Design review of the part built by this model. Coordinates are the model's own, in mm. A direction names the side the tool comes from. Round coordinates to 2 decimals unless told otherwise and drop trailing zeros. Loops run counter-clockwise (first coordinate to the right, second up) from the corner with the lowest first, then second, coordinate; pieces in that order, holes last. Notation, with made-up numbers: (39.25, -29.75) - (49.25, -29.75) arc R26 cw to (49.25, -3.75) - close; hole circle Ø3 at (31.25, 23.5). An arc over 180 degrees is marked (long way). Answer as CSV lines item,"result". Start each with the question number.
(1) For P1, Ø1.5, axis at x = 0.5, y = 2, coming from the +Z side; P2, Ø1, axis at x = 1.5, z = 3, coming from the +Y side; P3, Ø1.5, axis at x = 1.5, y = -1, coming from the -Z side, all flat-tipped, find the tip position at first contact; note any pin that passes through.
(2) Wall thickness on L1, parallel to X at y = -0.6, z = -2; L2, parallel to Y at x = -0.05, z = 2.25; L3, parallel to Z at x = 0, y = 1.55: over which ranges is each line inside the solid? List them lowest first.
(3) For faces 4 (the flat face through (0, 0, 5)), 5 (the cylindrical face through (-1.5, 0.07, 2.46)), list the 3-axis set-ups (+Z, -Z, +X, -X, +Y, -Y) from which the entire face can be reached by the end or side of a thin tool; tool diameter is ignored.
(4) Consider section C-C (z = 0.75). Give the boundary of the cut face in (x, y).
(5) Mouldability with a two-part tool opening along X and no side actions: class faces 1 (the cylindrical face through (-0.038, -0.035, -1.075)), 2 (the flat face through (0, -2.5, -0.9)), 3 (the cylindrical face through (1.75, -0.04, -0.61)) as released by +X, released by -X, zero draft, split by the parting line, or undercut.
(6) Consider section D-D (y = -1.25). Give the boundary of the cut face in (x, z).
(7) Consider section A-A (x = 0). Give the boundary of the cut face in (y, z).
(8) Consider section B-B (y = 0). Give the boundary of the cut face in (x, z), and give its area (4 significant figures).
from build123d import *

# Parameters (mm, degrees)
F1_DEPTH = 2.5
F2_R     = 1.5
F3_DEPTH = 5


with BuildPart() as f1:
    # F0 (on Front) → F1 (new body, symmetric)
    with BuildSketch(Plane.XZ):
        with BuildLine():
            ThreePointArc((-1.452369, -2.94996), (0, -1.07496), (1.452369, -2.94996))
            ThreePointArc((1.452369, -2.94996), (0, 0.42504), (-1.452369, -2.94996))
        make_face()
    extrude(amount=F1_DEPTH, both=True)

    # F2 (on Top) → F3 (join)
    with BuildSketch(Plane.XY):
        Circle(F2_R)
    extrude(amount=F3_DEPTH)


solid = f1.part
Determined:
1,P1,"stops at z = 5"
1,P2,"stops at y = 1.12"
1,P3,"stops at z = -2.95"
2,L1,"x = -1.95 to -1.39, 1.39 to 1.95"
2,L2,"y = -1.5 to 1.5"
2,L3,"z = -1.07 to 0.43"
3,face 4,"+Z, +X, -X, +Y, -Y"
3,face 5,"+Z"
4,outline,"circle Ø3 at (0, 0)"
5,face 1,"undercut"
5,face 2,"zero draft"
5,face 3,"split by the parting line"
6,outline,"(-1.45, -2.95) arc R1.5 cw (long way) to (1.45, -2.95) arc R2 ccw to (0.83, 0.25) - (0.83, 5) - (-0.83, 5) - (-0.83, 0.25) arc R2 ccw to start"
7,outline,"(-2.5, -1.07) - (2.5, -1.07) - (2.5, 0.43) - (1.5, 0.43) - (1.5, 5) - (-1.5, 5) - (-1.5, 0.43) - (-2.5, 0.43) - close"
8,outline,"(-1.5, 0) - (-1.23, 0) arc R2 ccw to (-1.45, -2.95) arc R1.5 cw (long way) to (1.45, -2.95) arc R2 ccw to (1.23, 0) - (1.5, 0) - (1.5, 5) - (-1.5, 5) - close"
8,area,"20.95 mm^2"
